Check sheet for the drawn part. Datum: minimum x, y, z corner. Units: mm. A direction names the side the tool comes from. Give positions to 0.01 mm unless a question says otherwise; leave off trailing zeros. Order: outer loops, then holes, each group sorted by start corner. A loop starts at its lowest first (then second) coordinate and runs counter-clockwise, first axis right, second up.
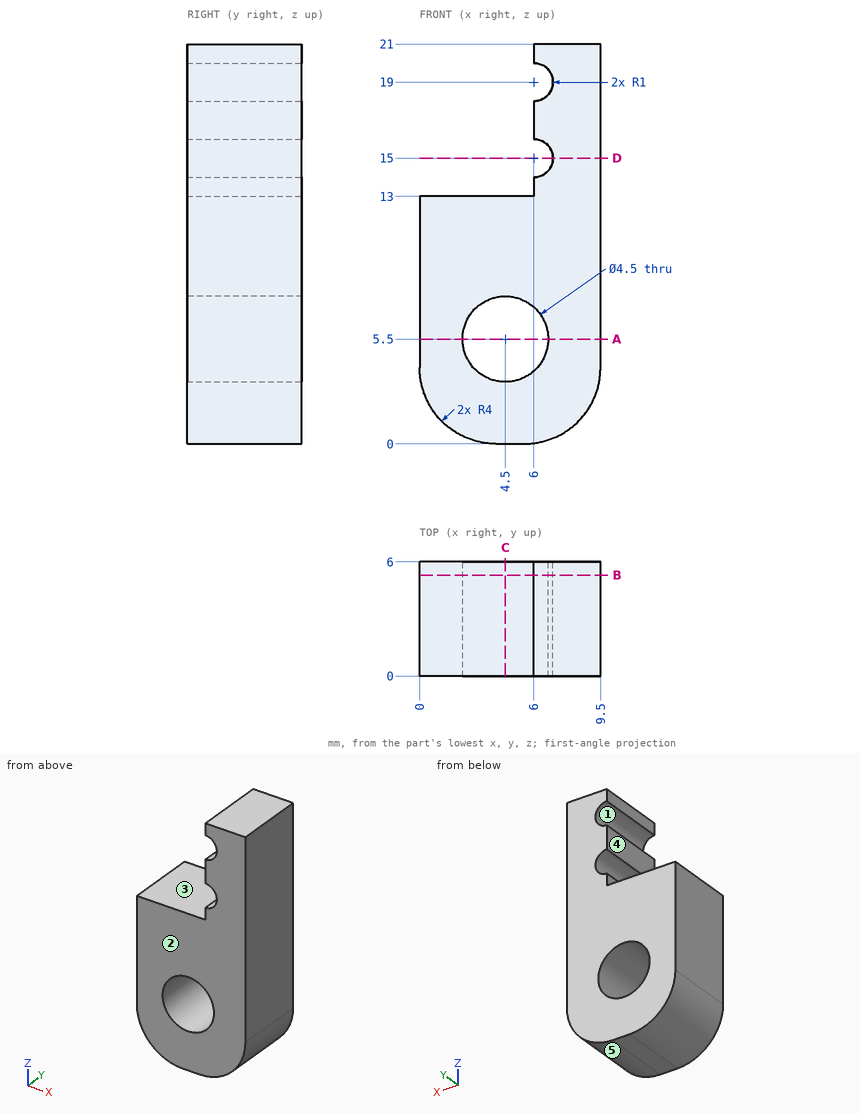
Item 1: Scan lines: L1, parallel to X at y = 3.95, z = 5.5; L2, parallel to X at y = 3.05, z = 19; L3, parallel to Z at x = 5.75, y = 3.05. Record each from-to range of solid material in increasing order.
Reported:
L1: x = 0 to 2.25, 6.75 to 9.5
L2: x = 7 to 9.5
L3: z = 0.01 to 3.63, 7.37 to 13
Item 2: Sectioned sample at B-B (y = 5.3). Enter the section's corners in (x, z).
Reported:
outline: (0, 4) arc R4 ccw to (4, 0) - (5.5, 0) arc R4 ccw to (9.5, 4) - (9.5, 21) - (6, 21) - (6, 20) arc R1 cw to (6, 18) - (6, 16) arc R1 cw to (6, 14) - (6, 13) - (0, 13) - close; hole circle Ø4.5 at (4.5, 5.5)
Item 3: Draft check along Z on the marked faces 1, 2 and 3. Enter one of: released by +Z, released by -Z, zero draft, split by the parting line, or undercut.
Reported:
face 1: undercut
face 2: zero draft
face 3: released by +Z
Item 4: Sectioned sample at A-A (z = 5.5). Enter the section's corners in (x, y).
Reported:
outline: (0, 0) - (2.25, 0) - (2.25, 6) - (0, 6) - close; (6.75, 0) - (9.5, 0) - (9.5, 6) - (6.75, 6) - close
Item 5: Set-up check for the marked faces 4 and 5: record each of +Z, -Z, +X, -X, +Y, -Y from which the full face is reachable in a straight line by a thin tool's end or side.
Reported:
face 4: +Z, -X, +Y, -Y
face 5: -Z, +X, +Y, -Y
Item 6: Sectioned sample at D-D (z = 15). Enter the section's corners in (x, y), and give its area (3 significant figures).
Reported:
outline: (7, 0) - (9.5, 0) - (9.5, 6) - (7, 6) - close
area: 15.0 mm2
Item 7: Gauge pin test, flat end, axial feed: pin 1 (2 mm diameter, centred on y = 1, z = 18, fed in from -X). Record the tip position at first contact, or that the pin passes through.
Reported:
pin 1: stops at x = 6
Item 8: Sectioned sample at C-C (x = 4.5). Enter the section's corners in (y, z).
Reported:
outline: (0, 0) - (6, 0) - (6, 3.25) - (0, 3.25) - close; (0, 7.75) - (6, 7.75) - (6, 13) - (0, 13) - close
